Study the drawing (mm; zero at the part's minimum x, y, z) and answer. A direction names the side the tool comes from. Give positions to 0.01 mm unless a question says otherwise; leave off trailing zeros. Order: outer loops, then holes, each group sorted by start corner. A loop starts at its lowest first (then second) coordinate and runs counter-clockwise, first axis right, second up.
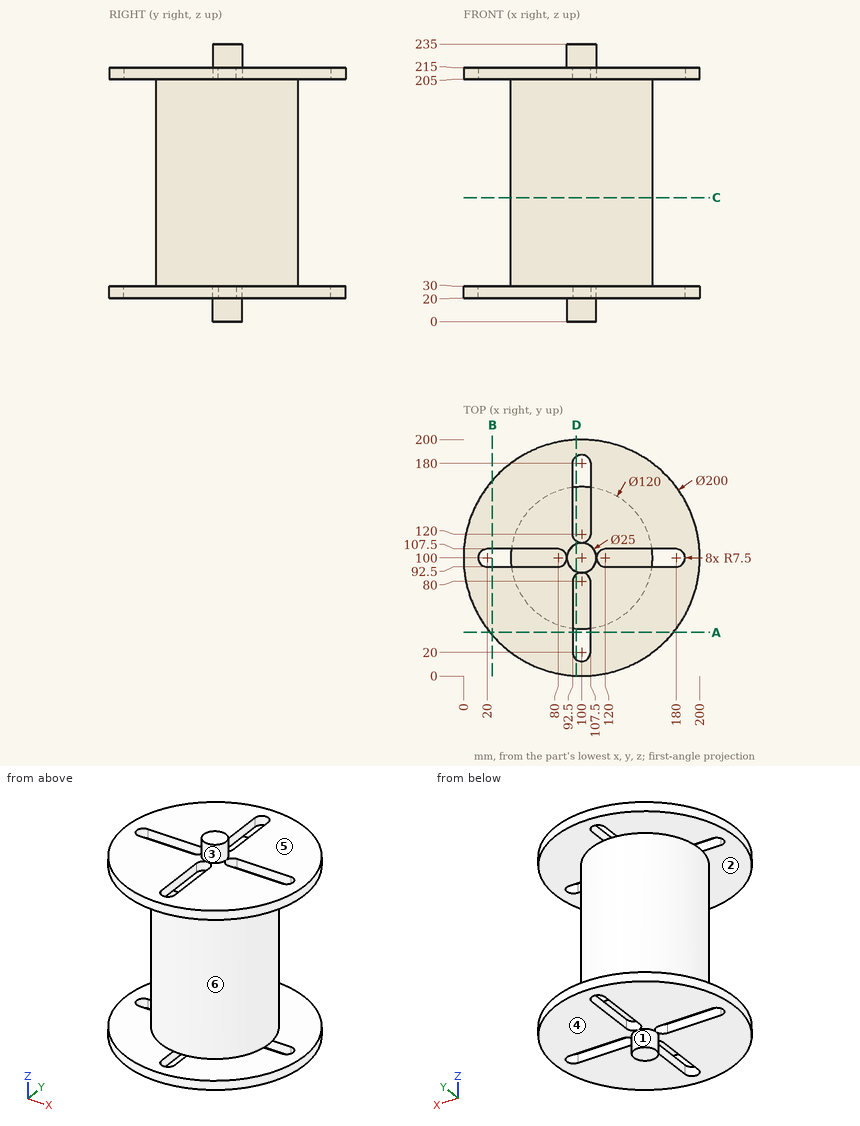
1) A tool of negligible diameter and unlimited length cuts with its end or side. For the marked faces 1 and 2, from which of +Z, -Z, +X, -X, +Y, -Y can it reach the whole face along a straight path? Write none if from no direction.
Geometry says:
face 1: -Z
face 2: none
2) Find section C-C (z = 105). Write down the section's boundary in (x, y), then the cut area to 3 significant figures.
Geometry says:
outline: circle Ø120 at (100, 100)
area: 11,300 mm2
3) Find section A-A (y = 37). Write down the section's boundary in (x, z), then the cut area to 3 significant figures.
Geometry says:
outline: (22.34, 20) - (92.5, 20) - (92.5, 30) - (22.34, 30) - close; (22.34, 205) - (92.5, 205) - (92.5, 215) - (22.34, 215) - close; (107.5, 20) - (177.66, 20) - (177.66, 30) - (107.5, 30) - close; (107.5, 205) - (177.66, 205) - (177.66, 215) - (107.5, 215) - close
area: 2,810 mm2
4) Straight lines are drawn through the part: probe 1 along Z at (x, y) = (56, 43); probe 2 along Z at (x, y) = (119.5, 71); probe 3 along Y at (x, z) = (55, 25). For each, find the intervals that lie inside material, in ascending order.
Geometry says:
probe 1: z = 20 to 30, 205 to 215
probe 2: z = 20 to 215
probe 3: y = 10.7 to 92.5, 107.5 to 189.3
5) Given P1, Ø4.5, axis at x = 143.5, y = 98, coming from the +Z side; P2, Ø8, axis at x = 127, z = 38.5, coming from the +Y side; P3, Ø8, axis at y = 49, z = 210.5, coming from the -X side, each flat-ended and moving along its own axis, determine where each tip first touches the part or whether it passes through.
Geometry says:
P1: stops at z = 205
P2: stops at y = 155.42
P3: stops at x = 11.73
6) Find section D-D (x = 95.5). Count the separate pieces of the cut face and the enclosed holes in it, then the cut area to 3 significant figures.
Geometry says:
separate pieces: 5
enclosed holes: 0
area: 23,000 mm2
7) Find section B-B (x = 24.5). Write down the section's boundary in (y, z), then the cut area to 3 significant figures.
Geometry says:
outline: (34.43, 20) - (92.5, 20) - (92.5, 30) - (34.43, 30) - close; (34.43, 205) - (92.5, 205) - (92.5, 215) - (34.43, 215) - close; (107.5, 20) - (165.57, 20) - (165.57, 30) - (107.5, 30) - close; (107.5, 205) - (165.57, 205) - (165.57, 215) - (107.5, 215) - close
area: 2,320 mm2
8) For a pull along Z with two mould halves and no side action, classify the marked faces 3, 4, 5 and 6 as +Z half, -Z half, draft (parallel to the pull), parting line (faces both ways), or undercut.
Geometry says:
face 3: draft
face 4: -Z half
face 5: +Z half
face 6: undercut
